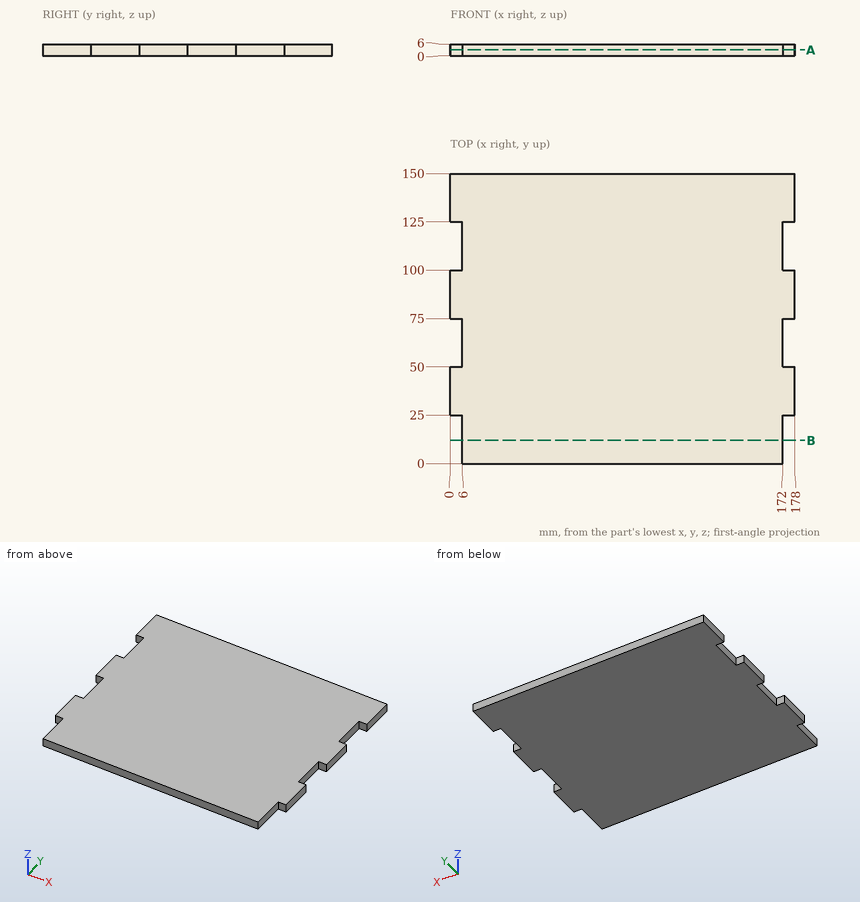
Input: dimensioned drawing with shaded views. Units: mm. Origin: part minimum x, y, z. Coordinates: 2 decimals unless noted, no trailing zeros. Loops run counter-clockwise (first coordinate to the right, second up) from the corner with the lowest first, then second, coordinate; pieces in that order, holes last. Notation, with made-up numbers: (14, 47.25) -> (20, 47.25) arc R13 ccw to (20, 63.25) -> close; hole circle Ø10 at (-3.5, 12). An arc over 180 degrees is marked (long way). One line per item, written item: value. Start each with the question number.
Q1. Contact query for flat-ended pins moving along their axis: P1, Ø3, axis at x = 4, z = 1.5, coming from the -Y side; P2, Ø5, axis at x = 55, y = 74, coming from the -Z side; P3, Ø1.8, axis at y = 115, z = 3.5, coming from the -X side. Output: stop coordinate, or through.
Q2. Section query B-B, the plane y = 12. Return the cut outline in (x, z), and give its area (3 significant figures).
Q3. Section query A-A, the plane z = 2.9. Return the cut outline in (x, y), and give its area (3 significant figures).
Q4. Line query: line 1 along X through (y, z) = (71.5, 5.05). Output: solid intervals per line, ascending.
Results:
1. P1: y = 25
1. P2: z = 0
1. P3: x = 6
2. outline: (6, 0) -> (172, 0) -> (172, 6) -> (6, 6) -> close
2. area: 996 mm^2
3. outline: (0, 25) -> (6, 25) -> (6, 0) -> (172, 0) -> (172, 25) -> (178, 25) -> (178, 50) -> (172, 50) -> (172, 75) -> (178, 75) -> (178, 100) -> (172, 100) -> (172, 125) -> (178, 125) -> (178, 150) -> (0, 150) -> (0, 125) -> (6, 125) -> (6, 100) -> (0, 100) -> (0, 75) -> (6, 75) -> (6, 50) -> (0, 50) -> close
3. area: 25,800 mm^2
4. line 1: 6 to 172
